Geometry: final body of the model. Coordinates: model frame, mm. Give positions to 0.01 mm unless a question says otherwise; leave off trailing zeros. Order: outer loops, then holes, each group sorted by start corner. A loop starts at its lowest first (then second) coordinate and runs counter-clockwise, first axis right, second up. Notation, with made-up numbers: M 89,52.5 L 141,52.5 A25 ccw 141,83.5 Z; hole C -3,-5.5 d3. An arc over 180 degrees is marked long. Write item = value, one per line. Start each with the question number.
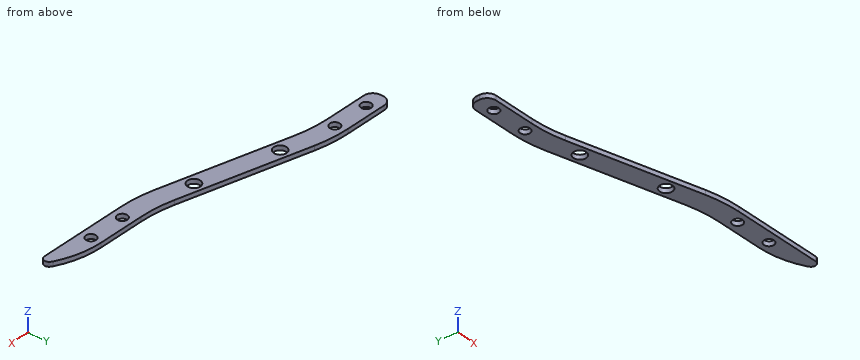
from build123d import *

# Parameters (mm, degrees)
SKETCH_2_R          = 1.1
EXTRUDE_1_DEPTH     = 1
SKETCH_4_R          = 1.4
CUT_EXTRUDE_1_DEPTH = 38.745650692


with BuildPart() as part:
    # 草图2 → 凸台-拉伸1 (new body)
    with BuildSketch(Plane.XY):
        with BuildLine():
            Line((9.2004412, -1.304787978), (-18.44790974, 5.804787978))
            ThreePointArc((-18.44790974, 5.804787978), (-22.15374848, 6.512758939), (-25.919140934, 6.75))
            Line((-25.919140934, 6.75), (-35.12373427, 6.75))
            ThreePointArc((-35.12373427, 6.75), (-36.537947832, 6.164213562), (-37.12373427, 4.75))
            Line((-37.12373427, 4.75), (-37.12373427, 4.25))
            ThreePointArc((-37.12373427, 4.25), (-36.537947832, 2.835786438), (-35.12373427, 2.25))
            Line((-35.12373427, 2.25), (-25.92398706, 2.25))
            ThreePointArc((-25.92398706, 2.25), (-22.153862686, 2.012159905), (-18.443517429, 1.302410814))
            Line((-18.443517429, 1.302410814), (9.149963579, -5.802410814))
            ThreePointArc((9.149963579, -5.802410814), (12.860308836, -6.512159905), (16.63043321, -6.75))
            Line((16.63043321, -6.75), (36.12373427, -6.75))
            ThreePointArc((36.12373427, -6.75), (37.035192863, -6.161391824), (36.873667496, -5.088486466))
            ThreePointArc((36.873667496, -5.088486466), (36.618179656, -4.845779883), (36.32405992, -4.651681705))
            ThreePointArc((36.32405992, -4.651681705), (31.722166726, -2.859714212), (26.821471158, -2.25))
            Line((26.821471158, -2.25), (16.671672394, -2.25))
            ThreePointArc((16.671672394, -2.25), (12.90627994, -2.012758939), (9.2004412, -1.304787978))
        make_face()
        with Locations((26.821471158, -4.5)):
            Circle(SKETCH_2_R, mode=Mode.SUBTRACT)
        with Locations((18.821471158, -4.5)):
            Circle(SKETCH_2_R, mode=Mode.SUBTRACT)
        with Locations((-25.12373427, 4.5)):
            Circle(SKETCH_2_R, mode=Mode.SUBTRACT)
        with Locations((-33.125142276, 4.5)):
            Circle(SKETCH_2_R, mode=Mode.SUBTRACT)
    extrude(amount=EXTRUDE_1_DEPTH)

    # 草图4 → 切除-拉伸1 (cut, through all)
    with BuildSketch(Plane.XY.offset(1)):
        with Locations((-13.6677648, 2.324207374)):
            Circle(SKETCH_4_R)
        with Locations((3.3322352, -2.049984423)):
            Circle(SKETCH_4_R)
    extrude(amount=-CUT_EXTRUDE_1_DEPTH, mode=Mode.SUBTRACT)


solid = part.part
1) Ray query, L1, parallel to Y at x = -33, z = 0.1; L2, parallel to Y at x = 33.5, z = 0.1; L3, parallel to Y at x = 18, z = 0.7. Return the intervals inside material, ascending.
2) Cut plane B-B (x = 30). Return loops of the section in (y, z).
3) Cut plane C-C (x = -11). Return loops of the section in (y, z), plus the area to 3 significant figures.
4) Pin query (flat end, axial travel): pin 1 Ø3 at (x, y) = (-21.5, 3) entering from -Z; pin 2 Ø0.5 at (x, z) = (-28.5, 0.5) entering from -Y. Return the tip coordinate at first contact, or that it passes through.
5) Cut plane A-A (z = 0.6). Return loops of the section in (x, y), plus the area to 3 significant figures.
Reply:
q1.L1 = 2.25 to 3.41, 5.59 to 6.75
q1.L2 = -6.75 to -3.4
q1.L3 = -6.75 to -5.23, -3.77 to -2.25
q2.outline = M -6.75,0 L -2.5,0 L -2.5,1 L -6.75,1 Z
q3.outline = M -0.61,0 L 3.89,0 L 3.89,1 L -0.61,1 Z
q3.area = 4.50 mm²
q4.pin_1 = 0
q4.pin_2 = 2.25
q5.outline = M -37.12,4.25 A2 ccw -35.12,2.25 L -25.92,2.25 A30 cw -18.44,1.3 L 9.15,-5.8 A30 ccw 16.63,-6.75 L 36.12,-6.75 A1 ccw 36.87,-5.09 A2 ccw 36.32,-4.65 A20 ccw 26.82,-2.25 L 16.67,-2.25 A30 cw 9.2,-1.3 L -18.45,5.8 A30 ccw -25.92,6.75 L -35.12,6.75 A2 ccw -37.12,4.75 Z; hole C -33.13,4.5 d2.2; hole C -25.12,4.5 d2.2; hole C -13.67,2.32 d2.8; hole C 3.33,-2.05 d2.8; hole C 18.82,-4.5 d2.2; hole C 26.82,-4.5 d2.2
q5.area = 295 mm²
